Check sheet for the modelled part. Datum: model origin and axes. Units: mm. A direction names the side the tool comes from. Give positions to 0.01 mm unless a question says otherwise; leave off trailing zeros. Order: outer loops, then holes, each group sorted by start corner. A loop starts at its lowest first (then second) coordinate and runs counter-clockwise, first axis right, second up. Notation, with made-up numbers: (-4, 41.5) -> (17, 41.5) arc R29 cw to (17, 80.5) -> close; hole circle Ø9 at (-18, 73). An arc over 180 degrees is marked (long way). One line per question, with ' | ' between items.
```python
from build123d import *

# Parameters (mm, degrees)
SKETCH_1_R          = 10
SKETCH_1_R_2        = 1.5
SKETCH_1_R_3        = 1
EXTRUDE_1_DEPTH     = 3
SKETCH_2_R          = 4.5
EXTRUDE_2_DEPTH     = 2
SKETCH_3_R          = 3
CUT_EXTRUDE_1_DEPTH = 3.5
SKETCH_4_R          = 1.5
CUT_EXTRUDE_2_DEPTH = 10


with BuildPart() as part:
    # 草图1 → 凸台-拉伸1 (new body)
    with BuildSketch(Plane.XY):
        Circle(SKETCH_1_R)
        Circle(SKETCH_1_R_2, mode=Mode.SUBTRACT)
        with Locations((0, 8)):
            Circle(SKETCH_1_R_3, mode=Mode.SUBTRACT)
        with Locations((5.656854249, 5.656854249)):
            Circle(SKETCH_1_R_3, mode=Mode.SUBTRACT)
        with Locations((8, 0)):
            Circle(SKETCH_1_R_3, mode=Mode.SUBTRACT)
        with Locations((5.656854249, -5.656854249)):
            Circle(SKETCH_1_R_3, mode=Mode.SUBTRACT)
        with Locations((0, -8)):
            Circle(SKETCH_1_R_3, mode=Mode.SUBTRACT)
        with Locations((-5.656854249, -5.656854249)):
            Circle(SKETCH_1_R_3, mode=Mode.SUBTRACT)
        with Locations((-8, 0)):
            Circle(SKETCH_1_R_3, mode=Mode.SUBTRACT)
        with Locations((-5.656854249, 5.656854249)):
            Circle(SKETCH_1_R_3, mode=Mode.SUBTRACT)
    extrude(amount=EXTRUDE_1_DEPTH)

    # 草图2 → 凸台-拉伸2 (add)
    with BuildSketch(Plane(origin=(0, 0, 0), x_dir=(-1, 0, 0), z_dir=(0, 0, -1))):
        with Locations(Location((0, 0, 0), (0, 0, 180))):
            Circle(SKETCH_2_R)
    extrude(amount=EXTRUDE_2_DEPTH)

    # 草图3 → 切除-拉伸1 (cut)
    with BuildSketch(Plane(origin=(0, 0, 3), x_dir=(-1, 0, 0), z_dir=(0, 0, -1))):
        Circle(SKETCH_3_R)
    extrude(amount=CUT_EXTRUDE_1_DEPTH, mode=Mode.SUBTRACT)

    # 草图4 → 切除-拉伸2 (cut)
    with BuildSketch(Plane(origin=(0, 0, -2), x_dir=(-1, 0, 0), z_dir=(0, 0, -1))):
        Circle(SKETCH_4_R)
    extrude(amount=-CUT_EXTRUDE_2_DEPTH, mode=Mode.SUBTRACT)


solid = part.part
```
Q1. Depth check by flat-ended pin: pin 1 Ø12 at (x, y) = (-6, -3.5) entering from -Z; pin 2 Ø1.6 at (x, y) = (-8, 0) entering from +Z; pin 3 Ø3 at (x, y) = (-5.66, -5.66) entering from -Z; pin 4 Ø3 at (x, z) = (-4.5, -0.5) entering from +Y. Enter the tip coordinate at first touch or a pass-through.
Result sheet:
pin 1: stops at z = -2 | pin 2: passes through | pin 3: stops at z = 0 | pin 4: stops at y = 9.51
Q2. Mould release check, pull along X, two halves, no side actions. Record for faces 1 (the face through (5.527, -4.665, 1.479)), 2 (the face through (-6.656, -5.613, 1.479)), 3 (the face through (2.1, 2.4, 3)), 4 (the face through (-2.17, -9.76, 1.48)): pulls with the +X half, pulls with the -X half, needs draft (parallel to the pull), parting line crosses it, or undercut.
Result sheet:
face 1: undercut | face 2: undercut | face 3: needs draft | face 4: parting line crosses it
Q3. Thickness scan on line 1 (X direction, y = 6, z = 2.3); line 2 (Y direction, x = -0.25, z = 0.3); line 3 (Y direction, x = 6.5, z = 1.15). Record the ranges inside material, lowest first.
Result sheet:
line 1: x = -8 to -6.6, -4.72 to 4.72, 6.6 to 8 | line 2: y = -10 to -8.97, -7.03 to -2.99, 2.99 to 7.03, 8.97 to 10 | line 3: y = -7.6 to -6.19, -5.12 to 5.12, 6.19 to 7.6
Q4. Section check D-D (y = -6). Enter the section's corners in (x, z).
Result sheet:
outline: (-8, 0) -> (-6.6, 0) -> (-6.6, 3) -> (-8, 3) -> close; (-4.72, 0) -> (4.72, 0) -> (4.72, 3) -> (-4.72, 3) -> close; (6.6, 0) -> (8, 0) -> (8, 3) -> (6.6, 3) -> close
Q5. Section check A-A (x = 0). Enter the section's corners in (y, z).
Result sheet:
outline: (-10, 0) -> (-9, 0) -> (-9, 3) -> (-10, 3) -> close; (-7, 0) -> (-4.5, 0) -> (-4.5, -2) -> (-1.5, -2) -> (-1.5, -0.5) -> (-3, -0.5) -> (-3, 3) -> (-7, 3) -> close; (1.5, -2) -> (4.5, -2) -> (4.5, 0) -> (7, 0) -> (7, 3) -> (3, 3) -> (3, -0.5) -> (1.5, -0.5) -> close; (9, 0) -> (10, 0) -> (10, 3) -> (9, 3) -> close
Q6. Access from +Z, -Z, +X, -X, +Y, -Y to the whole of each face (thin tool, end or side, straight path). Record for faces 5 (the face through (-5, 0, 0)), 6 (the face through (3, 0, 1)), 7 (the face through (0, 9, 1)).
Result sheet:
face 5: -Z | face 6: +Z | face 7: +Z, -Z
Q7. Section check C-C (x = -8). Enter the section's corners in (y, z).
Result sheet:
outline: (-6, 0) -> (-1, 0) -> (-1, 3) -> (-6, 3) -> close; (1, 0) -> (6, 0) -> (6, 3) -> (1, 3) -> close
